Read the model definition and answer for the solid it produces. Units are mm, in the model's axes. Give positions to 0.01 mm unless a question says otherwise; leave off trailing zeros. Write each loop counter-clockwise with the first axis right and the second up, starting at its lowest first coordinate (ties: lowest second). Pieces come first, ordered by that corner, then holes. Notation, with made-up numbers: (36, 72) - (43, 72) arc R35 ccw to (43, 111) - close; hole circle Ø4 at (-15.75, 67.25). An arc over 180 degrees is marked (long way). Answer as CSV lines item,"result".
```python
from build123d import *
from OCP.BRepFilletAPI import BRepFilletAPI_MakeChamfer

# Parameters (mm, degrees)
BOSS_EXTRUDE1_DEPTH = 2.5
FILLET1_R           = 0.2
SKETCH2_W           = 0.6
SKETCH2_H           = 0.6
BOSS_EXTRUDE2_DEPTH = 5.81
CHAMFER1_SIZE       = 0.1
CHAMFER1_SIZE2      = 0.214450692


with BuildPart() as part:
    # Sketch1 → Boss-Extrude1 (new body)
    with BuildSketch(Plane(origin=(0, 0, 0), x_dir=(1, 0, 0), z_dir=(0, 1, 0))):
        Polygon((1.25, 0.75), (1.5, 0.75), (1.5, -0.75), (1.25, -0.75), (1.25, -1.25), (-1.25, -1.25), (-1.25, -0.75), (-1.5, -0.75), (-1.5, 0.75), (-1.25, 0.75), (-1.25, 1.25), (1.25, 1.25), align=None)
    extrude(amount=BOSS_EXTRUDE1_DEPTH)

    # Fillet1
    fillet1_edges = [part.edges().sort_by_distance(p)[0] for p in [
        (-1.5, 2.5, 0),
        (0, 0, -1.25),
        (1.25, 0, -1),
        (1.375, 0, -0.75),
        (1.5, 0, 0),
        (1.375, 0, 0.75),
        (1.25, 0, 1),
        (-1.375, 2.5, 0.75),
        (0, 0, 1.25),
        (-1.25, 0, 1),
        (-1.375, 0, 0.75),
        (-1.5, 0, 0),
        (-1.375, 0, -0.75),
        (-1.25, 0, -1),
        (-1.25, 2.5, 1),
        (0, 2.5, 1.25),
        (-1.25, 1.25, -1.25),
        (1.25, 1.25, -1.25),
        (1.5, 1.25, -0.75),
        (1.5, 1.25, 0.75),
        (1.25, 1.25, 1.25),
        (-1.25, 1.25, 1.25),
        (-1.5, 1.25, 0.75),
        (-1.5, 1.25, -0.75),
        (1.25, 2.5, 1),
        (1.375, 2.5, 0.75),
        (1.5, 2.5, 0),
        (1.375, 2.5, -0.75),
        (1.25, 2.5, -1),
        (0, 2.5, -1.25),
        (-1.25, 2.5, -1),
        (-1.375, 2.5, -0.75),
    ]]
    fillet(fillet1_edges, radius=FILLET1_R)

    # Sketch2 → Boss-Extrude2 (add, symmetric)
    with BuildSketch(Plane(origin=(0, 2.5, 0), x_dir=(1, 0, 0), z_dir=(0, 1, 0))):
        Rectangle(SKETCH2_W, SKETCH2_H)
    extrude(amount=BOSS_EXTRUDE2_DEPTH, both=True)

    # Chamfer1: one chamfer whose edges measure the first distance from different faces: ONE call of the kernel's chamfer builder (chamfer() names one face for all edges)
    chamfer1_edges_1 = [part.edges().sort_by_distance(p)[0] for p in [
        (-0.3, -3.31, 0),
        (0, -3.31, 0.3),
        (0.3, -3.31, 0),
        (0, -3.31, -0.3),
    ]]
    chamfer1_side_1 = [part.faces().sort_by_distance(p)[0] for p in [
        (0, -3.31, 0),
    ]]
    chamfer1_edges_2 = [part.edges().sort_by_distance(p)[0] for p in [
        (-0.3, 8.31, 0),
    ]]
    chamfer1_side_2 = [part.faces().sort_by_distance(p)[0] for p in [
        (-0.3, 5.405, 0),
    ]]
    chamfer1_edges_3 = [part.edges().sort_by_distance(p)[0] for p in [
        (0, 8.31, 0.3),
    ]]
    chamfer1_side_3 = [part.faces().sort_by_distance(p)[0] for p in [
        (0, 5.405, 0.3),
    ]]
    chamfer1_edges_4 = [part.edges().sort_by_distance(p)[0] for p in [
        (0.3, 8.31, 0),
    ]]
    chamfer1_side_4 = [part.faces().sort_by_distance(p)[0] for p in [
        (0.3, 5.405, 0),
    ]]
    chamfer1_edges_5 = [part.edges().sort_by_distance(p)[0] for p in [
        (0, 8.31, -0.3),
    ]]
    chamfer1_side_5 = [part.faces().sort_by_distance(p)[0] for p in [
        (0, 5.405, -0.3),
    ]]
    chamfer1 = BRepFilletAPI_MakeChamfer(part.part.solid().wrapped)
    for e in chamfer1_edges_1:
        chamfer1.Add(CHAMFER1_SIZE, CHAMFER1_SIZE2, e.wrapped, chamfer1_side_1[0].wrapped)  # the first distance lies on this face
    for e in chamfer1_edges_2:
        chamfer1.Add(CHAMFER1_SIZE, CHAMFER1_SIZE2, e.wrapped, chamfer1_side_2[0].wrapped)  # the first distance lies on this face
    for e in chamfer1_edges_3:
        chamfer1.Add(CHAMFER1_SIZE, CHAMFER1_SIZE2, e.wrapped, chamfer1_side_3[0].wrapped)  # the first distance lies on this face
    for e in chamfer1_edges_4:
        chamfer1.Add(CHAMFER1_SIZE, CHAMFER1_SIZE2, e.wrapped, chamfer1_side_4[0].wrapped)  # the first distance lies on this face
    for e in chamfer1_edges_5:
        chamfer1.Add(CHAMFER1_SIZE, CHAMFER1_SIZE2, e.wrapped, chamfer1_side_5[0].wrapped)  # the first distance lies on this face
    add(Compound.cast(chamfer1.Shape()), mode=Mode.REPLACE)


solid = part.part
```
(1) A cutting plane is placed at A-A (z = 0.4). Write down the section's boundary in (x, y), and give its area (3 significant figures).
Worked out:
outline,"(-1.5, 0.2) arc R0.2 ccw to (-1.3, 0) - (1.3, 0) arc R0.2 ccw to (1.5, 0.2) - (1.5, 2.3) arc R0.2 ccw to (1.3, 2.5) - (-1.3, 2.5) arc R0.2 ccw to (-1.5, 2.3) - close"
area,"7.47 mm^2"
(2) Each of these flat-tipped pins is pushed along its axis until it touches: P1, Ø0.7, axis at x = 0, y = -1.5, coming from the -Z side; P2, Ø0.5, axis at y = -1.5, z = 0, coming from the -X side; P3, Ø1, axis at x = 1, z = 0.5, coming from the +Y side. Where does it stop, or does it pass through?
Worked out:
P1,"stops at z = -0.3"
P2,"stops at x = -0.3"
P3,"stops at y = 2.5"
(3) Find the intervals of material crossed by L1, parallel to Y at x = 0.35, z = 0.7; L2, parallel to Z at x = 0.05, y = 6.75, in increasing order.
Worked out:
L1,"y = 0 to 2.5"
L2,"z = -0.3 to 0.3"
(4) A cutting plane is placed at D-D (y = 5.25). Write down the section's boundary in (x, z), and give its area (3 significant figures).
Worked out:
outline,"(-0.3, -0.3) - (0.3, -0.3) - (0.3, 0.3) - (-0.3, 0.3) - close"
area,"0.360 mm^2"
(5) A cutting plane is placed at C-C (x = 0.5). Write down the section's boundary in (y, z).
Worked out:
outline,"(0, -1.05) arc R0.2 ccw to (0.2, -1.25) - (2.3, -1.25) arc R0.2 ccw to (2.5, -1.05) - (2.5, 1.05) arc R0.2 ccw to (2.3, 1.25) - (0.2, 1.25) arc R0.2 ccw to (0, 1.05) - close"
(6) A cutting plane is placed at B-B (y = 1.25). Write down the section's boundary in (x, z).
Worked out:
outline,"(-1.5, -0.55) arc R0.2 ccw to (-1.3, -0.75) - (-1.25, -0.75) - (-1.25, -1.05) arc R0.2 ccw to (-1.05, -1.25) - (1.05, -1.25) arc R0.2 ccw to (1.25, -1.05) - (1.25, -0.75) - (1.3, -0.75) arc R0.2 ccw to (1.5, -0.55) - (1.5, 0.55) arc R0.2 ccw to (1.3, 0.75) - (1.25, 0.75) - (1.25, 1.05) arc R0.2 ccw to (1.05, 1.25) - (-1.05, 1.25) arc R0.2 ccw to (-1.25, 1.05) - (-1.25, 0.75) - (-1.3, 0.75) arc R0.2 ccw to (-1.5, 0.55) - close"
